Part model, mm, in its own coordinate system. Coordinates: 2 decimals unless noted, no trailing zeros. Loops run counter-clockwise (first coordinate to the right, second up) from the corner with the lowest first, then second, coordinate; pieces in that order, holes last. Notation, with made-up numbers: (31.5, 76) - (57.5, 76) arc R27 ccw to (57.5, 103) - close; hole circle Ø10 at (82, 20). An arc over 180 degrees is marked (long way). Use a Markdown table: item, result. Add a question column.
1) Drop flat-ended pins along their axis: P1, Ø0.9, axis at x = 2, z = 40.5, coming from the -Y side; P2, Ø0.9, axis at x = 1.5, y = 2.5, coming from the +Z side; P3, Ø1.5, axis at x = 2, z = -73.5, coming from the -Y side; P4, Ø2, axis at y = 5.5, z = 30.5, coming from the -X side. Give the stop position or say it passes through.
2) Band-saw the part on C-C (y = 0). Give the cut face in (x, z).
3) Band-saw the part on D-D (z = 30.5). Give the cut face in (x, y).
4) Band-saw the part on B-B (x = 0.6). Give the number of separate pieces and of enclosed holes in the cut face, plus the area to 3 significant figures.
5) Band-saw the part on A-A (z = -22). Give the cut face in (x, y), plus the area to 3 significant figures.
6) Probe probe 1 along Y at (x, z) = (0.1, 19.5); probe 2 along Y at (x, z) = (0.8, 60.5); probe 3 along Y at (x, z) = (1.45, 38.5). List the from-to ranges inside material, lowest first. Write a range as [from, to].
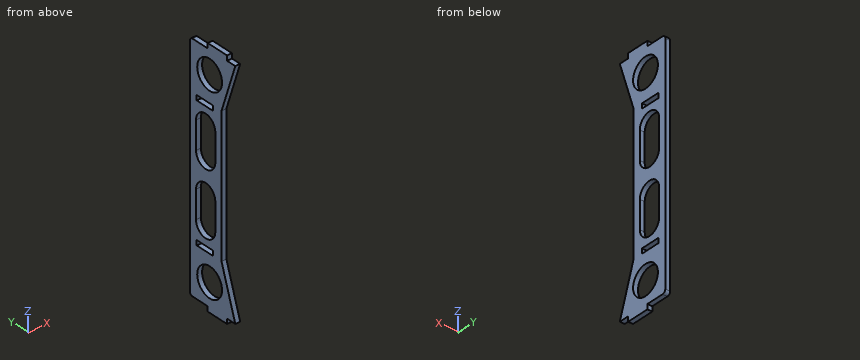
from build123d import *

# Parameters (mm, degrees)
SKETCH1_W           = 144
SKETCH1_H           = 23
BOSS_EXTRUDE1_DEPTH = 3
FILLET1_R           = 2
BOSS_EXTRUDE2_DEPTH = 3
SKETCH3_W           = 3
SKETCH3_H           = 14
BOSS_EXTRUDE3_DEPTH = 3
SKETCH4_R           = 9
SKETCH4_W           = 3
SKETCH4_H           = 12
CUT_EXTRUDE1_DEPTH  = 10


with BuildPart() as part:
    # Sketch1 → Boss-Extrude1 (new body)
    with BuildSketch(Plane(origin=(0, 0, 0), x_dir=(0, 0, -1), z_dir=(1, 0, 0))):
        Rectangle(SKETCH1_W, SKETCH1_H)
    extrude(amount=BOSS_EXTRUDE1_DEPTH)

    # Fillet1
    fillet1_edges = [part.edges().sort_by_distance(p)[0] for p in [
        (1.5, 11.5, 72),
        (1.5, 11.5, -72),
    ]]
    fillet(fillet1_edges, radius=FILLET1_R)

    # Sketch2 → Boss-Extrude2 (add)
    with BuildSketch(Plane(origin=(3, 0, 0), x_dir=(0, 0, -1), z_dir=(1, 0, 0))):
        Polygon((-72, -11.5), (-72, -21.5), (-42, -11.5), align=None)
        Polygon((72, -11.5), (72, -21.5), (42, -11.5), align=None)
    extrude(amount=-BOSS_EXTRUDE2_DEPTH)

    # Sketch3 → Boss-Extrude3 (add)
    with BuildSketch(Plane(origin=(3, 0, 0), x_dir=(0, 0, -1), z_dir=(1, 0, 0))):
        with Locations((-73.5, -8.5)):
            Rectangle(SKETCH3_W, SKETCH3_H)
        with Locations((73.5, -8.5)):
            Rectangle(SKETCH3_W, SKETCH3_H)
    extrude(amount=-BOSS_EXTRUDE3_DEPTH)

    # Sketch4 → Cut-Extrude1 (cut)
    with BuildSketch(Plane(origin=(3, 0, 0), x_dir=(0, 0, -1), z_dir=(1, 0, 0))):
        with Locations((-57.942503038, -2.875250136)):
            Circle(SKETCH4_R)
        with Locations((57.942503038, -2.875250136)):
            Circle(SKETCH4_R)
        with Locations((-40.5, 0.5)):
            Rectangle(SKETCH4_W, SKETCH4_H)
        with Locations((40.5, 0.5)):
            Rectangle(SKETCH4_W, SKETCH4_H)
        with BuildLine():
            Line((-27.851450915, 7), (-10.851450915, 7))
            ThreePointArc((-10.851450915, 7), (-3.851450915, 0), (-10.851450915, -7))
            Line((-10.851450915, -7), (-27.851450915, -7))
            ThreePointArc((-27.851450915, -7), (-34.851450915, 0), (-27.851450915, 7))
        make_face()
        with BuildLine():
            Line((27.851450915, 7), (10.851450915, 7))
            ThreePointArc((10.851450915, 7), (3.851450915, 0), (10.851450915, -7))
            Line((10.851450915, -7), (27.851450915, -7))
            ThreePointArc((27.851450915, -7), (34.851450915, 0), (27.851450915, 7))
        make_face()
    extrude(amount=-CUT_EXTRUDE1_DEPTH, mode=Mode.SUBTRACT)


solid = part.part
Answer block:
| question | item | result |
|---|---|---|
| 1 | P1 | y = -11.5 |
| 1 | P2 | z = 72 |
| 1 | P3 | y = -15.5 |
| 1 | P4 | x = 0 |
| 2 | outline | (0, -72) - (3, -72) - (3, -66.47) - (0, -66.47) - close; (0, -49.41) - (3, -49.41) - (3, -42) - (0, -42) - close; (0, -39) - (3, -39) - (3, -34.85) - (0, -34.85) - close; (0, -3.85) - (3, -3.85) - (3, 3.85) - (0, 3.85) - close; (0, 34.85) - (3, 34.85) - (3, 39) - (0, 39) - close; (0, 42) - (3, 42) - (3, 49.41) - (0, 49.41) - close; (0, 66.47) - (3, 66.47) - (3, 72) - (0, 72) - close |
| 3 | outline | (0, -11.5) - (3, -11.5) - (3, -6.48) - (0, -6.48) - close; (0, 6.48) - (3, 6.48) - (3, 11.5) - (0, 11.5) - close |
| 4 | separate pieces | 1 |
| 4 | enclosed holes | 6 |
| 4 | area | 2,330 mm2 |
| 5 | outline | (0, -11.5) - (3, -11.5) - (3, -7) - (0, -7) - close; (0, 7) - (3, 7) - (3, 11.5) - (0, 11.5) - close |
| 5 | area | 27.0 mm2 |
| 6 | probe 1 | [-11.5, -7], [7, 11.5] |
| 6 | probe 2 | [-17.67, -11.5], [5.75, 11.5] |
| 6 | probe 3 | [-11.5, 11.5] |
